Read the model definition and answer for the solid it produces. Units are mm, in the model's axes. Give positions to 0.01 mm unless a question says otherwise; leave off trailing zeros. Loops run counter-clockwise (first coordinate to the right, second up) from the corner with the lowest first, then second, coordinate; pieces in that order, holes last. Notation, with made-up numbers: (-28, 41.5) - (14, 41.5) arc R23 ccw to (14, 53.5) - close; hole circle Ø4 at (-7, 78.25). An arc over 180 degrees is marked (long way). Write each question's results on one line, items separated by ' | '. Start each with the question number.
Q1. The part is cut by section A-A, the plane x = -36. Write down the section's boundary in (y, z), plus the area to 3 significant figures.
Q2. Find the intervals of material crossed by line 1 (Z direction, x = -32.5, y = 2.35); line 2 (X direction, y = 0.7, z = -33); line 3 (Z direction, x = -41, y = 2.45), in increasing order. Write a range as from..to.
Q3. The part is cut by section B-B, the plane z = -9.5. Write down the section's boundary in (x, y).
Q4. Given pin 1 (6 mm diameter, centred on x = 12.5, z = 3.5, fed in from -Y); pin 2 (0.8 mm diameter, centred on y = 1, z = -45, fed in from -X); pin 3 (0.8 mm diameter, centred on x = 47, y = 1.5, fed in from -Z), each flat-ended and moving along its own axis, determine where each tip first touches the part or whether it passes through.
```python
from build123d import *

# Parameters (mm, degrees)
SKETCH1_W           = 90
SKETCH1_H           = 20
SKETCH1_W_2         = 4.5
SKETCH1_H_2         = 8.2
SKETCH1_W_3         = 62
SKETCH1_H_3         = 3.6
SKETCH1_H_4         = 40
BOSS_EXTRUDE1_DEPTH = 2.5


with BuildPart() as part:
    # Sketch1 → Boss-Extrude1 (new body)
    with BuildSketch(Plane(origin=(0, 0, 0), x_dir=(1, 0, 0), z_dir=(0, 1, 0))):
        with Locations((0, 50)):
            Rectangle(SKETCH1_W, SKETCH1_H)
        Polygon((-45, 40), (-45, 31.8), (-40, 31.8), (-40, 34), (-31, 34), (-31, 31.8), (31, 31.8), (31, 34), (40, 34), (40, 31.8), (45, 31.8), (45, 40), align=None)
        with Locations((-47.25, 35.9)):
            Rectangle(SKETCH1_W_2, SKETCH1_H_2)
        with Locations((-47.25, 24.1)):
            Rectangle(SKETCH1_W_2, SKETCH1_H_2)
        Polygon((-45, 28.2), (-45, 20), (45, 20), (45, 28.2), (40, 28.2), (40, 26), (31, 26), (31, 28.2), (-31, 28.2), (-31, 26), (-40, 26), (-40, 28.2), align=None)
        with Locations((0, 30)):
            Rectangle(SKETCH1_W_3, SKETCH1_H_3)
        Rectangle(SKETCH1_W, SKETCH1_H_4)
        Polygon((-45, -20), (-45, -28.2), (-40, -28.2), (-40, -26), (-31, -26), (-31, -28.2), (31, -28.2), (31, -26), (40, -26), (40, -28.2), (45, -28.2), (45, -20), align=None)
        with Locations((-47.25, -24.1)):
            Rectangle(SKETCH1_W_2, SKETCH1_H_2)
        with Locations((-47.25, -35.9)):
            Rectangle(SKETCH1_W_2, SKETCH1_H_2)
        Polygon((-45, -31.8), (-45, -40), (45, -40), (45, -31.8), (40, -31.8), (40, -34), (31, -34), (31, -31.8), (-31, -31.8), (-31, -34), (-40, -34), (-40, -31.8), align=None)
        with Locations((0, -30)):
            Rectangle(SKETCH1_W_3, SKETCH1_H_3)
        with Locations((47.25, -24.1)):
            Rectangle(SKETCH1_W_2, SKETCH1_H_2)
        with Locations((47.25, -35.9)):
            Rectangle(SKETCH1_W_2, SKETCH1_H_2)
        with Locations((47.25, 24.1)):
            Rectangle(SKETCH1_W_2, SKETCH1_H_2)
        with Locations((47.25, 35.9)):
            Rectangle(SKETCH1_W_2, SKETCH1_H_2)
        with Locations((0, -50)):
            Rectangle(SKETCH1_W, SKETCH1_H)
    extrude(amount=BOSS_EXTRUDE1_DEPTH)


solid = part.part
```
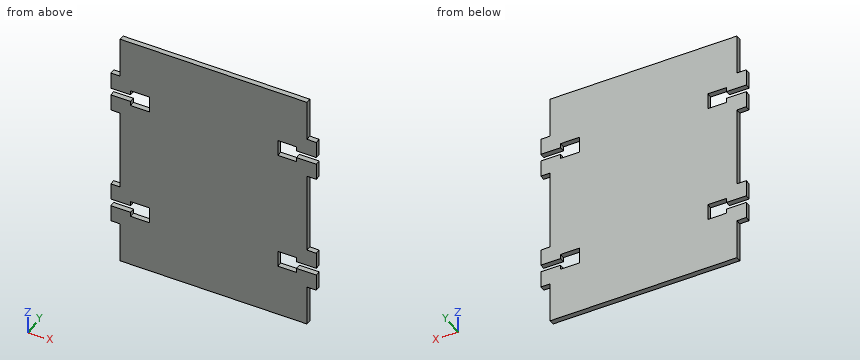
Check sheet entries:
1) outline: (0, -60) - (2.5, -60) - (2.5, -34) - (0, -34) - close; (0, -26) - (2.5, -26) - (2.5, 26) - (0, 26) - close; (0, 34) - (2.5, 34) - (2.5, 60) - (0, 60) - close | area: 260 mm^2
2) line 1: z = -60..-34, -26..26, 34..60 | line 2: x = -49.5..-40, -31..31, 40..49.5 | line 3: z = -60..-31.8, -28.2..28.2, 31.8..60
3) outline: (-45, 0) - (45, 0) - (45, 2.5) - (-45, 2.5) - close
4) pin 1: stops at y = 0 | pin 2: stops at x = -45 | pin 3: stops at z = -40
